```python
from build123d import *

# Parameters (mm, degrees)
SKETCH1_R                = 46.99
SKETCH1_R_2              = 3.175
SKETCH1_R_3              = 9.75
SKETCH1_R_4              = 4
BOSS_EXTRUDE1_DEPTH      = 17
CUT_EXTRUDE2_DEPTH       = 69.593878736
BOSS_EXTRUDE2_DEPTH      = 5.08
BOSS_EXTRUDE2_DEPTH_BACK = 17
SKETCH7_R                = 27.9
SKETCH7_R_2              = 24
CUT_EXTRUDE3_START       = -3.81
SKETCH8_R                = 24
CUT_EXTRUDE3_DEPTH       = 3.81


with BuildPart() as part:
    # Sketch1 → Boss-Extrude1 (new body)
    with BuildSketch(Plane.XY):
        Circle(SKETCH1_R)
        with Locations((0, 15.875)):
            Circle(SKETCH1_R_2, mode=Mode.SUBTRACT)
        Circle(SKETCH1_R_3, mode=Mode.SUBTRACT)
        with Locations((0, 37.500000057)):
            Circle(SKETCH1_R_4, mode=Mode.SUBTRACT)
        with Locations((-32.475952658, 18.750000086)):
            Circle(SKETCH1_R_4, mode=Mode.SUBTRACT)
        with Locations((-32.475952757, -18.749999915)):
            Circle(SKETCH1_R_4, mode=Mode.SUBTRACT)
        with Locations((32.475952658, 18.750000086)):
            Circle(SKETCH1_R_4, mode=Mode.SUBTRACT)
        with Locations((32.475952362, -18.749999914)):
            Circle(SKETCH1_R_4, mode=Mode.SUBTRACT)
        with Locations((-1.97e-07, -37.500000057)):
            Circle(SKETCH1_R_4, mode=Mode.SUBTRACT)
        with Locations((13.748153285, 7.9375)):
            Circle(SKETCH1_R_2, mode=Mode.SUBTRACT)
        with Locations((13.748153285, -7.9375)):
            Circle(SKETCH1_R_2, mode=Mode.SUBTRACT)
        with Locations((0, -15.875)):
            Circle(SKETCH1_R_2, mode=Mode.SUBTRACT)
        with Locations((-13.748153285, -7.9375)):
            Circle(SKETCH1_R_2, mode=Mode.SUBTRACT)
        with Locations((-13.748153285, 7.9375)):
            Circle(SKETCH1_R_2, mode=Mode.SUBTRACT)
    extrude(amount=BOSS_EXTRUDE1_DEPTH)

    # Sketch3 → Cut-Extrude2 (cut, through all)
    with BuildSketch(Plane.XY.offset(17)):
        with BuildLine():
            add(Edge.make_bspline(
                [(0, 46.99), (-14.204157194, 45.847251077), (-7.045904013, 28.257565433), (-13.97, 24.196749782)],
                knots=[0, 0, 0, 0, 1, 1, 1, 1], degree=3))
            ThreePointArc((0, 46.99), (-23.495, 40.694533724), (-40.694533724, 23.495))
            add(Edge.make_bspline(
                [(-40.694533724, 23.495), (-32.602805529, 35.224786508), (-20.948817508, 20.230714585), (-13.97, 24.196749782)],
                knots=[0, 0, 0, 0, 1, 1, 1, 1], degree=3))
        make_face()
        with BuildLine():
            ThreePointArc((40.694533724, 23.495), (23.495, 40.694533724), (0, 46.99))
            add(Edge.make_bspline(
                [(0, 46.99), (14.204157194, 45.847251077), (7.045904013, 28.257565433), (13.97, 24.196749782)],
                knots=[0, 0, 0, 0, 1, 1, 1, 1], degree=3))
            add(Edge.make_bspline(
                [(40.694533724, 23.495), (32.602805529, 35.224786508), (20.948817508, 20.230714585), (13.97, 24.196749782)],
                knots=[0, 0, 0, 0, 1, 1, 1, 1], degree=3))
        make_face()
        with BuildLine():
            ThreePointArc((46.99, 0), (45.388854577, 12.161906929), (40.694533724, 23.495))
            add(Edge.make_bspline(
                [(40.694533724, 23.495), (46.806962724, 10.622464569), (27.994721521, 8.026850849), (27.94, 0)],
                knots=[0, 0, 0, 0, 1, 1, 1, 1], degree=3))
            add(Edge.make_bspline(
                [(40.694533724, -23.495), (46.806962724, -10.622464569), (27.994721521, -8.026850849), (27.94, 0)],
                knots=[0, 0, 0, 0, 1, 1, 1, 1], degree=3))
            ThreePointArc((40.694533724, -23.495), (45.388854577, -12.161906929), (46.99, 0))
        make_face()
        with BuildLine():
            ThreePointArc((0, -46.99), (23.495, -40.694533724), (40.694533724, -23.495))
            add(Edge.make_bspline(
                [(40.694533724, -23.495), (32.602805529, -35.224786508), (20.948817508, -20.230714585), (13.97, -24.196749782)],
                knots=[0, 0, 0, 0, 1, 1, 1, 1], degree=3))
            add(Edge.make_bspline(
                [(0, -46.99), (14.204157194, -45.847251077), (7.045904013, -28.257565433), (13.97, -24.196749782)],
                knots=[0, 0, 0, 0, 1, 1, 1, 1], degree=3))
        make_face()
        with BuildLine():
            add(Edge.make_bspline(
                [(-40.694533724, -23.495), (-32.602805529, -35.224786508), (-20.948817508, -20.230714585), (-13.97, -24.196749782)],
                knots=[0, 0, 0, 0, 1, 1, 1, 1], degree=3))
            ThreePointArc((-40.694533724, -23.495), (-23.495, -40.694533724), (0, -46.99))
            add(Edge.make_bspline(
                [(0, -46.99), (-14.204157194, -45.847251077), (-7.045904013, -28.257565433), (-13.97, -24.196749782)],
                knots=[0, 0, 0, 0, 1, 1, 1, 1], degree=3))
        make_face()
        with BuildLine():
            add(Edge.make_bspline(
                [(-40.694533724, 23.495), (-46.806962724, 10.622464569), (-27.994721521, 8.026850849), (-27.94, 0)],
                knots=[0, 0, 0, 0, 1, 1, 1, 1], degree=3))
            ThreePointArc((-40.694533724, 23.495), (-46.99, 0), (-40.694533724, -23.495))
            add(Edge.make_bspline(
                [(-40.694533724, -23.495), (-46.806962724, -10.622464569), (-27.994721521, -8.026850849), (-27.94, 0)],
                knots=[0, 0, 0, 0, 1, 1, 1, 1], degree=3))
        make_face()
    extrude(amount=-CUT_EXTRUDE2_DEPTH, mode=Mode.SUBTRACT)

    # Sketch7 → Boss-Extrude2 (add, two sides: drawn at the far end of the back side and taken through both)
    with BuildSketch(Plane.XY.offset(17).offset(-BOSS_EXTRUDE2_DEPTH_BACK)):
        Circle(SKETCH7_R)
        Circle(SKETCH7_R_2, mode=Mode.SUBTRACT)
    extrude(amount=BOSS_EXTRUDE2_DEPTH + BOSS_EXTRUDE2_DEPTH_BACK)

    # Sketch8 → Cut-Extrude3 (cut)
    with BuildSketch(Plane.XY.offset(17).offset(CUT_EXTRUDE3_START)):
        Circle(SKETCH8_R)
    extrude(amount=CUT_EXTRUDE3_DEPTH, mode=Mode.SUBTRACT)


solid = part.part
```
Geometry check sheet. Reference: the model listing, model coordinates, mm. A direction names the side the tool comes from. Round coordinates to 2 decimals unless told otherwise and drop trailing zeros. Order: outer loops, then holes, each group sorted by start corner. A loop starts at its lowest first (then second) coordinate and runs counter-clockwise, first axis right, second up. Notation, with made-up numbers: (-37.75, 4) -> (-20.75, 4) arc R12 cw to (-20.75, 10) -> close; hole circle Ø2 at (38.5, -5). An arc over 180 degrees is marked (long way). Return JSON: item names as keys, results as strings. Group by question number.
Q1. Release check for a two-part mould opening along X. For faces 3 (the flat face through (-24.5, -13.7, 17)), 4 (the cylindrical face through (36.29, 19.95, 8.38)), 5 (the cylindrical face through (-6.048, -27.237, 19.504)) record: released by +X, released by -X, zero draft, split by the parting line, or undercut.
Q2. Material ranges on probe 1 along Y at (x, z) = (0, 8.5); probe 2 along X at (y, z) = (-0.5, 19); probe 3 along Y at (x, z) = (2.5, 16.5), recorded low to high. Write a range as from..to.
Q3. Gauge pin test, flat ends, axial feed: pin 1 (5.5 mm diameter, centred on x = -13.75, y = 7.94, fed in from -Z); pin 2 (8 mm diameter, centred on y = -3, z = 9, fed in from +X); pin 3 (8.5 mm diameter, centred on x = 13.75, y = 7.94, fed in from +Z); pin 4 (12 mm diameter, centred on y = 2, z = 6, fed in from -X). Record the tip position at first contact, or that the pin passes through.
Q4. Section check A-A, the plane z = 20.5. Record the boundary of the cut face in (x, y).
Q5. Tool access check on faces 1 (the flat face through (0, -10, 13.19)), 2 (the flat face through (-1, 11, 0)). Record the directions out of +Z, -Z, +X, -X, +Y, -Y that give a thin tool (end or side, any length) a straight path to the whole face; none if there is none.
Q6. Section check B-B, the plane x = -1.5. Count the separate pieces of the cut face and the enclosed holes in it, plus the area to 3 significant figures.
Numbers:
{
 "1": {"face 3": "zero draft", "face 4": "undercut", "face 5": "split by the parting line"},
 "2": {"probe 1": "-46.99..-41.5, -33.5..-19.05, -12.7..-9.75, 9.75..12.7, 19.05..33.5, 41.5..46.99", "probe 2": "-27.9..-23.99, 23.99..27.9", "probe 3": "-46.57..-40.62, -34.38..-23.87, 23.87..34.38, 40.62..46.57"},
 "3": {"pin 1": "through", "pin 2": "x = 32.88", "pin 3": "z = 13.19", "pin 4": "x = -34.17"},
 "4": {"outline": "circle Ø55.8 at (0, 0); hole circle Ø48 at (0, 0)"},
 "5": {"face 1": "+Z", "face 2": "-Z, +X, -X, +Y, -Y"},
 "6": {"separate pieces": "6", "enclosed holes": "0", "area": "794 mm^2"}
}
